Autodesk Inventor part; units mm, degrees
ref_plane "YZ Plane" through (0, 0, 0) normal (1, 0, 0) x (0, 1, 0)
ref_plane "XZ Plane" through (0, 0, 0) normal (0, 1, 0) x (-1, 0, 0)
ref_plane "XY Plane" through (0, 0, 0) normal (0, 0, 1) x (1, 0, 0)
sketch "Sketch1" plane through (0, 0, 0) normal (0, 1, 0) x (-1, 0, 0)
  line L0 (0, 0) -> (20, 0)
  line L1 (20, 0) -> (20, -54)
  line L2 (20, -54) -> (0, -54)
  line L3 (0, -54) -> (0, 0)
  line L4 (20, -27) -> (0, -27)
  line L5 (-17, -17) -> (37, -17)
  line L6 (37, -17) -> (37, -37)
  line L7 (37, -37) -> (-17, -37)
  line L8 (-17, -37) -> (-17, -17)
  line L9 (-17, -17) -> (37, -37) construction
  line L10 (37, -17) -> (-17, -37) construction
  point P0 (10, -27)
  point P1 (0, -17)
  point P2 (0, -37)
  point P3 (20, -37)
  point P4 (20, -17)
  dimension "d0" = 20
  dimension "d1" = 54
  dimension "d2" = 54
  dimension "d3" = 20
extrude "Extrusion1" add sketch "Sketch1" along normal blind 2.5
sketch "Sketch2" plane through (0, 2.5, 0) normal (0, 1, 0) x (1, 0, 0)
  line L0 (-20, 0) -> (0, 0)
  line L1 (0, 0) -> (0, 17)
  line L2 (-20, 0) -> (0, 0)
  line L3 (0, 0) -> (0, 2)
  line L4 (0, 2) -> (-20, 2)
  line L5 (-20, 2) -> (-20, 0)
  dimension "d6" = 2
extrude "Extrusion2" add sketch "Sketch2" along normal blind 5
sketch "Sketch3" plane through (0, 2.5, 0) normal (0, 1, 0) x (1, 0, 0)
  line L0 (0, 2) -> (0, 17)
  line L1 (-20, 37) -> (0, 17)
  line L2 (0, 17) -> (-20, 17)
  line L3 (-20, 17) -> (0, 37)
  point P0 (0, 0)
  point P1 (-10, 27)
pattern_circular "Circular Pattern1" count 4 over 360 about axis through (-10, 2.5, -27) along (0, 1, 0) of "Extrusion2"
fillet "Fillet1" radius 2.25 4 edges at (-10, 0, 0) (-37, 0, -27) (-10, 0, -54) (17, 0, -27)
sketch "Sketch4" plane through (-20, 0, -17) normal (-1, 0, 0) x (0, 0, 1)
  point P0 (17, 0)
Part model, mm, in its own coordinate system. A direction names the side the tool comes from. Round coordinates to 2 decimals unless told otherwise and drop trailing zeros. Loops run counter-clockwise (first coordinate to the right, second up) from the corner with the lowest first, then second, coordinate; pieces in that order, holes last. Notation, with made-up numbers: (11, 56.25) -> (67, 56.25) arc R20 ccw to (67, 85.25) -> close; hole circle Ø6 at (-22, -25.5). An arc over 180 degrees is marked (long way). Use CSV: the item, a comma, the result in double quotes. Start each with the question number.
1) Which spindle directions (+Z, -Z, +X, -X, +Y, -Y) get a long thin tool onto all of the face, cutting with end or side? Do faces 5 (the flat face through (-10, 5, -52)), 6 (the flat face through (10, 2, -17)), 7 (the flat face through (-30, 2, -37)). Say none if no direction does.
2) Cut at A-A, the plane y = 5.5. Write the cut outline in (x, z), plus the area to 3 significant figures.
3) Cut at B-B, the plane x = -4. Write the cut outline in (y, z), plus the area to 3 significant figures.
4) Cut at D-D, the plane z = -8. Write the cut outline in (x, y), plus the area to 3 significant figures.
5) Drop flat-ended pins along their axis: P1, Ø4, axis at x = -13.5, y = 5.5, coming from the +Z side; P2, Ø2, axis at x = 10, z = -26, coming from the +Y side; P3, Ø2, axis at y = 4.5, z = -43, coming from the +X side; P4, Ø2, axis at y = 2, z = -48, coming from the -X side. Give the stop position or say it passes through.
6) Pull direction X, two halves, no side cores. Call faces 1 (the flat face through (-10, 2.5, -27)), 2 (the flat face through (11, 2, -37)), 3 (the flat face through (17, 5, -27)), 4 (the flat face through (-20, 2, -7)): +X half, -X half, draft (parallel to the pull), parting line (faces both ways), or undercut.
7) Wall check: L1, parallel to X at y = 6.75, z = -23; L2, parallel to Y at x = -24.5, z = -21; L3, parallel to Z at x = -1.5, y = 6. Give the ranges that are in metal, low to high. Write a range as [from, to].
8) Cut at C-C, the plane z = -33.5. Write the cut outline in (x, y).
Determined:
1,face 5,"+X, -X, +Y"
1,face 6,"+Z, +X, +Y, -Y"
1,face 7,"-Z, -X, +Y, -Y"
2,outline,"(-37, -37) -> (-35, -37) -> (-35, -17) -> (-37, -17) -> close; (-20, -54) -> (0, -54) -> (0, -52) -> (-20, -52) -> close; (-20, -2) -> (0, -2) -> (0, 0) -> (-20, 0) -> close; (15, -37) -> (17, -37) -> (17, -17) -> (15, -17) -> close"
2,area,"160 mm2"
3,outline,"(0, -51.75) arc R2.25 ccw to (2.25, -54) -> (7.5, -54) -> (7.5, -52) -> (2.5, -52) -> (2.5, -2) -> (7.5, -2) -> (7.5, 0) -> (2.25, 0) arc R2.25 ccw to (0, -2.25) -> close"
3,area,"153 mm2"
4,outline,"(-20, 0) -> (0, 0) -> (0, 2.5) -> (-20, 2.5) -> close"
4,area,"50.0 mm2"
5,P1,"stops at z = 0"
5,P2,"stops at y = 2.5"
5,P3,"passes through"
5,P4,"stops at x = -20"
6,face 1,"undercut"
6,face 2,"draft"
6,face 3,"+X half"
6,face 4,"-X half"
7,L1,"x = [-37, -35], [15, 17]"
7,L2,"y = [0, 2.5]"
7,L3,"z = [-54, -52], [-2, 0]"
8,outline,"(-37, 2.25) arc R2.25 ccw to (-34.75, 0) -> (14.75, 0) arc R2.25 ccw to (17, 2.25) -> (17, 7.5) -> (15, 7.5) -> (15, 2.5) -> (-35, 2.5) -> (-35, 7.5) -> (-37, 7.5) -> close"
